```python
from build123d import *

# Parameters (mm, degrees)
F2_W     = 200
F2_H     = 120
F3_DEPTH = 63.2
F4_T     = -1.6
F5_W     = 1.6
F5_H     = 1.6
F5_H_2   = 22.2
F5_H_3   = 93
F5_W_2   = 91.4
F6_DEPTH = 61.6


with BuildPart() as f3:
    # F2 (on Top) → F3 (new body)
    with BuildSketch(Plane.XY):
        with Locations((74.1047750609, 38.4864358604)):
            Rectangle(F2_W, F2_H)
    extrude(amount=F3_DEPTH)

    # F4
    f4_openings = [f3.faces().sort_by_distance(p)[0] for p in [
        (74.104775, 38.486436, 63.2),
    ]]
    offset(amount=F4_T, openings=f4_openings)

    # F5 (on face) → F6 (join, through all)
    with BuildSketch(Plane.XY.offset(1.6)):
        with Locations((67.9047750609, 3.0864358604)):
            Rectangle(F5_W, F5_H)
        with Locations((67.9047750609, -8.8135641396)):
            Rectangle(F5_W, F5_H_2)
        Polygon((113.1492195054, 3.8864358604), (111.5492195054, 3.8864358604), (68.7047750609, 3.8864358604), (68.7047750609, 2.2864358604), (172.5047750609, 2.2864358604), (172.5047750609, 3.8864358604), align=None)
        with Locations((67.9047750609, 50.3864358604)):
            Rectangle(F5_W, F5_H_3)
        with Locations((21.4047750609, 3.0864358604)):
            Rectangle(F5_W_2, F5_H)
        with Locations((112.3492195054, 50.3864358604)):
            Rectangle(F5_W, F5_H_3)
    extrude(amount=F6_DEPTH)


solid = f3.part
```
Design review of the part built by this model. Coordinates are the model's own, in mm. A direction names the side the tool comes from. Coordinates: 2 decimals unless noted, no trailing zeros. Order: outer loops, then holes, each group sorted by start corner. A loop starts at its lowest first (then second) coordinate and runs counter-clockwise, first axis right, second up. Notation, with made-up numbers: (-22, 17) - (-18, 17) arc R27 cw to (-18, 52) - close; hole circle Ø7 at (66, 39). An arc over 180 degrees is marked (long way). Answer in a Markdown table with one row per item.
(1) Clearance check with flat-ended pins moving along their axes: pin 1 (1.5 mm diameter, centred on x = 129, y = 45, fed in from +Z); pin 2 (6 mm diameter, centred on x = 44, y = 80, fed in from -Z). State where each tip first meets the part, or that it passes through.
Checked values:
| item | result |
|---|---|
| pin 1 | z = 1.6 |
| pin 2 | z = 0 |
(2) Consider section C-C on y = 66.5. State the section outline as (x, z) points, plus the area to 3 significant figures.
Checked values:
| item | result |
|---|---|
| outline | (-25.9, 0) - (174.1, 0) - (174.1, 63.2) - (172.5, 63.2) - (172.5, 1.6) - (113.15, 1.6) - (113.15, 63.2) - (111.55, 63.2) - (111.55, 1.6) - (68.7, 1.6) - (68.7, 63.2) - (67.1, 63.2) - (67.1, 1.6) - (-24.3, 1.6) - (-24.3, 63.2) - (-25.9, 63.2) - close |
| area | 714 mm^2 |
(3) Consider section B-B on x = 55. State the section outline as (y, z) points.
Checked values:
| item | result |
|---|---|
| outline | (-21.51, 0) - (98.49, 0) - (98.49, 63.2) - (96.89, 63.2) - (96.89, 1.6) - (3.89, 1.6) - (3.89, 63.2) - (2.29, 63.2) - (2.29, 1.6) - (-19.91, 1.6) - (-19.91, 63.2) - (-21.51, 63.2) - close |
(4) For faces 1 (the flat face through (-25.895, 38, 31)), 2 (the flat face through (21, 96.886, 32)), list the 3-axis set-ups (+Z, -Z, +X, -X, +Y, -Y) from which the entire face can be reached by the end or side of a thin tool; tool diameter is ignored.
Checked values:
| item | result |
|---|---|
| face 1 | +Z, -Z, -X, +Y, -Y |
| face 2 | +Z |
(5) The part is to be moulded in two halves that separate along Y. For faces 3 (the flat face through (174.105, 38, 31)), 4 (the flat face through (142, 51, 1.6)), say which applies: released by +Y, released by -Y, zero draft, split by the parting line, or undercut.
Checked values:
| item | result |
|---|---|
| face 3 | zero draft |
| face 4 | undercut |
(6) Consider section D-D on y = -12. State the section outline as (x, z) points.
Checked values:
| item | result |
|---|---|
| outline | (-25.9, 0) - (174.1, 0) - (174.1, 63.2) - (172.5, 63.2) - (172.5, 1.6) - (68.7, 1.6) - (68.7, 63.2) - (67.1, 63.2) - (67.1, 1.6) - (-24.3, 1.6) - (-24.3, 63.2) - (-25.9, 63.2) - close |
(7) Wall thickness on line 1 along Y through (x, z) = (115, 47); line 2 along X through (y, z) = (-14.5, 33.5); line 3 along X through (y, z) = (23, 42): over which ranges is each line inside the solid? List them lowest first. Write a range as from..to.
Checked values:
| item | result |
|---|---|
| line 1 | -21.51..-19.91, 2.29..3.89, 96.89..98.49 |
| line 2 | -25.9..-24.3, 67.1..68.7, 172.5..174.1 |
| line 3 | -25.9..-24.3, 67.1..68.7, 111.55..113.15, 172.5..174.1 |
(8) Consider section A-A on z = 56. State the section outline as (x, y) points.
Checked values:
| item | result |
|---|---|
| outline | (-25.9, -21.51) - (174.1, -21.51) - (174.1, 98.49) - (-25.9, 98.49) - close; hole (-24.3, -19.91) - (67.1, -19.91) - (67.1, 2.29) - (-24.3, 2.29) - close; hole (-24.3, 3.89) - (67.1, 3.89) - (67.1, 96.89) - (-24.3, 96.89) - close; hole (68.7, -19.91) - (172.5, -19.91) - (172.5, 2.29) - (68.7, 2.29) - close; hole (68.7, 3.89) - (111.55, 3.89) - (111.55, 96.89) - (68.7, 96.89) - close; hole (113.15, 3.89) - (172.5, 3.89) - (172.5, 96.89) - (113.15, 96.89) - close |
